Input: part model. Units: mm. Frame: model coordinates. A direction names the side the tool comes from. Give positions to 0.01 mm unless a question says otherwise; leave off trailing zeros. Order: outer loops, then holes, each group sorted by start corner. A loop starts at its lowest first (then second) coordinate and runs counter-clockwise, first axis right, second up. Notation, with made-up numbers: M -2.5,44 L 46.5,44 A12 cw 46.5,48 Z; hole C -16.75,26 d3. An arc over 180 degrees is marked long. Use a Markdown table: item, result.
from build123d import *

# Parameters (mm, degrees)
SKETCH025_R             = 2
PAD015_DEPTH            = 52
POCKET009_DEPTH         = 60
SKETCH045_R             = 2
PAD026_DEPTH            = 25
LINEARPATTERN_COUNT     = 2
LINEARPATTERN_PITCH     = 25
FILLET005_R             = 24
FILLET006_R             = 6
BODY003_PLACEMENT_ANGLE = 180


with BuildPart() as part:
    # Sketch025 → Pad015 (new body)
    with BuildSketch(Plane.XZ):
        with BuildLine():
            ThreePointArc((-12.7279264704, -12.7279176523), (12.7279198568, -12.7279242659), (12.7279220614, 12.7279220614))
            Line((12.7279220614, 12.7279220614), (-14.605821279, 40.061665402))
            Line((-14.605821279, 40.061665402), (-147.231723, 40.061665402))
            Line((-147.231723, 40.061665402), (-147.231723, 3.061665402))
            Line((-147.231723, 3.061665402), (-28.5174940448, 3.061665402))
            Line((-12.7279264704, -12.7279176523), (-28.5174940448, 3.061665402))
        make_face()
        Circle(SKETCH025_R, mode=Mode.SUBTRACT)
    extrude(amount=PAD015_DEPTH)

    # Sketch026 (on Face5 of Pad015) → Pocket009 (cut)
    with BuildSketch(Plane(origin=(0, 0, -20.938334598), x_dir=(1, 0, 0), z_dir=(0, 0, -1))):
        with BuildLine():
            ThreePointArc((-121, 51), (-146, 26), (-121, 1))
            Line((-121, 1), (79, 1))
            ThreePointArc((79, 1), (104, 26), (79, 51))
            Line((-121, 51), (79, 51))
        make_face()
    extrude(amount=-POCKET009_DEPTH, mode=Mode.SUBTRACT)

    # Sketch045 (on Face13 of Pocket009) → Pad026 (join)
    with BuildSketch(Plane(origin=(0, 0, 39.061665402), x_dir=(1, 0, 0), z_dir=(0, 0, -1))):
        with BuildLine():
            Line((-47, 1), (-47, 5))
            ThreePointArc((-47, 5), (-50, 8), (-53, 5))
            Line((-53, 1), (-53, 5))
            Line((-47, 1), (-53, 1))
        make_face()
        with Locations((-50, 5)):
            Circle(SKETCH045_R, mode=Mode.SUBTRACT)
        with BuildLine():
            Line((-47, 51), (-47, 47))
            ThreePointArc((-53, 47), (-50, 44), (-47, 47))
            Line((-53, 51), (-53, 47))
            Line((-47, 51), (-53, 51))
        make_face()
        with Locations((-50, 47)):
            Circle(SKETCH045_R, mode=Mode.SUBTRACT)
    pad026 = extrude(amount=PAD026_DEPTH)

    # LinearPattern: Pad026 ×2
    with Locations(*[(-i * LINEARPATTERN_PITCH, 0, 0) for i in range(1, LINEARPATTERN_COUNT)]):
        add(pad026)

    # Fillet005
    fillet005_edges = [part.edges().sort_by_distance(p)[0] for p in [
        (-147.231723, 0, 21.561665),
        (-147.231723, -52, 21.561665),
    ]]
    fillet(fillet005_edges, radius=FILLET005_R)

    # Fillet006
    fillet006_edges = [part.edges().sort_by_distance(p)[0] for p in [
        (-68.918772, 0, 40.061665),
        (-140.202286, -7.029437, 40.061665),
        (-147.231723, -26, 40.061665),
        (-140.202286, -44.970563, 40.061665),
        (-68.918772, -52, 40.061665),
        (-146, -26, 39.061665),
        (-99.5, -51, 39.061665),
        (-62.5, -51, 39.061665),
        (-30.302911, -51, 39.061665),
        (-30.302911, -1, 39.061665),
        (-62.5, -1, 39.061665),
        (-99.5, -1, 39.061665),
    ]]
    fillet(fillet006_edges, radius=FILLET006_R)


with BuildPart() as part_1:
    # Body003 placement: moved
    add(part.part.moved(Location((0, -1, 0))).rotate(Axis((0, -1, 0), (0, 0, 1)), BODY003_PLACEMENT_ANGLE))


solid = part_1.part
1) First-contact query: pin 1 Ø5 at (x, y) = (75, 46) entering from +Z; pin 2 Ø1.2 at (x, y) = (51, 46.5) entering from -Z; pin 3 Ø8 at (y, z) = (6, 19.5) entering from -X; pin 4 Ø2 at (y, z) = (47.5, 32.5) entering from +X. Flat tips, straight axial feed; report the tip coordinate or a pass-through.
Response values:
| item | result |
|---|---|
| pin 1 | stops at z = 40.06 |
| pin 2 | stops at z = 39.06 |
| pin 3 | stops at x = 47 |
| pin 4 | stops at x = 137.22 |
2) Cut plane D-D on z = 19.5. State how many separate pieces and enclosed holes the cut face has, and give its area (3 significant figures).
Response values:
| item | result |
|---|---|
| separate pieces | 1 |
| enclosed holes | 4 |
| area | 491 mm² |
3) Cut plane A-A on x = 89. Return loops of the section in (y, z).
Response values:
| item | result |
|---|---|
| outline | M -1,3.06 L 0,3.06 L 0,33.06 A6 cw 6,39.06 L 44,39.06 A6 cw 50,33.06 L 50,3.06 L 51,3.06 L 51,34.06 A6 ccw 45,40.06 L 5,40.06 A6 ccw -1,34.06 Z |
4) Mould query, pull axis X, two halves, no side actions, for faces 1 (the face through (145.52, 25.03, 38.26)), 2 (the face through (-12.445, -0.507, -13.005)), 3 (the face through (47, 48, 27)), 4 (the face through (145.994, 25.55, 17.852)). Classes: released by +X, released by -X, zero draft, split by the parting line, or undercut.
Response values:
| item | result |
|---|---|
| face 1 | released by +X |
| face 2 | split by the parting line |
| face 3 | released by -X |
| face 4 | undercut |
5) Material intervals for line 1 (Y direction, x = 50, z = 29); line 2 (Y direction, x = 100, z = 4); line 3 (Z direction, x = 77.5, y = 10.5), sorted ascending. Write a range as from..to.
Response values:
| item | result |
|---|---|
| line 1 | y = -1..2, 6..7, 43..44, 48..51 |
| line 2 | y = -1..0, 50..51 |
| line 3 | z = 39.06..40.06 |
6) Cut plane C-C on x = 0. Return loops of the section in (y, z), and give its area (3 significant figures).
Response values:
| item | result |
|---|---|
| outline | M -1,-18 L 0,-18 L 0,-2 L -1,-2 Z; M -1,2 L 0,2 L 0,25.46 L -1,25.46 Z; M 50,-18 L 51,-18 L 51,-2 L 50,-2 Z; M 50,2 L 51,2 L 51,25.46 L 50,25.46 Z |
| area | 78.9 mm² |
7) Reachability of faces 5 (the face through (-0.923, 50.493, -1.774)), 6 (the face through (50, 43, 27)) from +Z, -Z, +X, -X, +Y, -Y: full face, straight path, thin tool, end or side. Return the list, or none.
Response values:
| item | result |
|---|---|
| face 5 | +Y, -Y |
| face 6 | -Z |
8) Cut plane B-B on z = -6. Return loops of the section in (x, y).
Response values:
| item | result |
|---|---|
| outline | M -16.97,-1 L 19.46,-1 L 19.46,0 L -16.97,0 Z; M -16.97,50 L 19.46,50 L 19.46,51 L -16.97,51 Z |
